Source: three-view drawing plus pictorial views. Frame: mm from the lowest corner of the part. Give positions to 0.01 mm unless a question says otherwise; leave off trailing zeros. Loops run counter-clockwise (first coordinate to the right, second up) from the corner with the lowest first, then second, coordinate; pieces in that order, holes last.
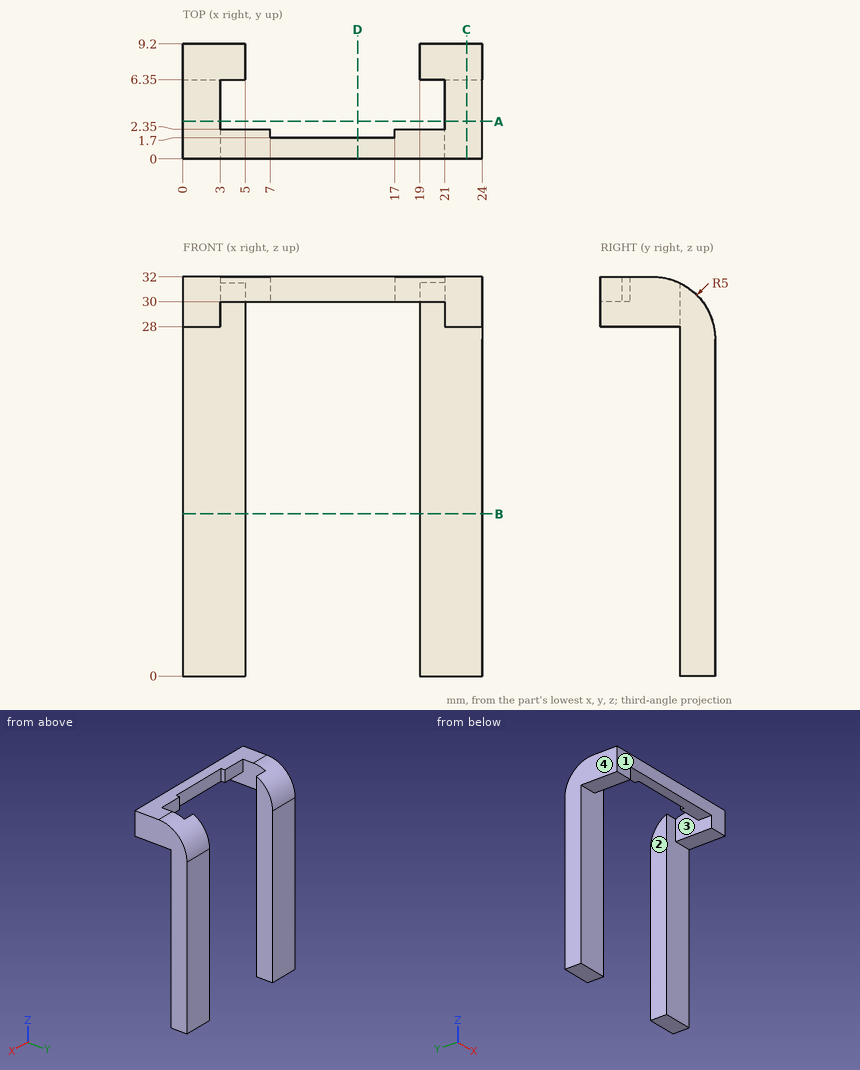
Q1. Section query B-B, the plane z = 13. Return loops of the section in (x, y).
Q2. Mould query, pull axis X, two halves, no side actions, for the marked faces 1, 2, 3 and 4. Classes: +X half, -X half, draft (parallel to the pull), parting line (faces both ways), or undercut.
Q3. Section query D-D, the plane x = 14. Return loops of the section in (y, z), and give its area (3 significant figures).
Q4. Section query A-A, the plane y = 3. Return loops of the section in (x, z).
Q5. Material intervals for probe 1 along X at (y, z) = (8.5, 12.5); probe 2 along Z at (x, y) = (22.5, 3); probe 3 along Y at (x, z) = (1, 17), sorted ascending.
Q6. Pin query (flat end, axial travel): pin 1 Ø2 at (x, z) = (4, 30.5) entering from +Y; pin 2 Ø5 at (x, y) = (20.5, 7) entering from +Z; pin 3 Ø1 at (x, z) = (19, 31.5) entering from +Y; pin 4 Ø4.5 at (y, z) = (4.5, 29.5) entering from -X. Return the tip coordinate at first contact, or that it passes through.
Q7. Section query C-C, the plane x = 22.75. Return loops of the section in (y, z).
Resolved:
1. outline: (0, 6.35) - (5, 6.35) - (5, 9.2) - (0, 9.2) - close; (19, 6.35) - (24, 6.35) - (24, 9.2) - (19, 9.2) - close
2. face 1: draft
2. face 2: undercut
2. face 3: undercut
2. face 4: -X half
3. outline: (0, 30) - (1.7, 30) - (1.7, 32) - (0, 32) - close
3. area: 3.40 mm2
4. outline: (0, 28) - (3, 28) - (3, 32) - (0, 32) - close; (21, 28) - (24, 28) - (24, 32) - (21, 32) - close
5. probe 1: x = 0 to 5, 19 to 24
5. probe 2: z = 28 to 32
5. probe 3: y = 6.35 to 9.2
6. pin 1: stops at y = 8.53
6. pin 2: stops at z = 31.99
6. pin 3: stops at y = 7.2
6. pin 4: stops at x = 0
7. outline: (0, 28) - (6.35, 28) - (6.35, 0) - (9.2, 0) - (9.2, 27) arc R5 ccw to (4.2, 32) - (0, 32) - close
